Could you check a few things on this model? Use its own coordinates, in mm. Face numbers are marked on the shaded views. A direction names the side the tool comes from. Give positions to 0.01 mm unless a question says otherwise; leave off trailing zeros. Write each loop counter-clockwise with the first axis right and the second up, starting at its lowest first coordinate (ties: lowest second). Pieces come first, ordered by that corner, then holes. Notation, with made-up numbers: M 21,32 L 43,32 A20 cw 43,48 Z; hole C 40.5,22 d2. An arc over 180 degrees is marked long. Answer as a JSON object with one key per item and string values. Group by question number.
Autodesk Inventor part; units mm, degrees
ref_plane "YZ Plane" through (0, 0, 0) normal (1, 0, 0) x (0, 1, 0)
ref_plane "XZ Plane" through (0, 0, 0) normal (0, 1, 0) x (-1, 0, 0)
ref_plane "XY Plane" through (0, 0, 0) normal (0, 0, 1) x (1, 0, 0)
sketch "Skizze1" plane through (0, 0, 0) normal (0, 0, 1) x (1, 0, 0)
  line L0 (-14, 0) -> (14, 0)
  line L1 (0, -14) -> (0, 14)
  circle A0 centre (0, 0) radius 7.5
  circle A1 centre (0, 0) radius 10
  dimension "d0" = 15
  dimension "d1" = 20
extrude "Extrusion1" add sketch "Skizze1" along normal mid plane 5 contours A0 L1 A1 L0 | L0 A1 L1 A0 | A0 L0 A1 L1 | L1 A1 L0 A0
sketch "Skizze2" plane through (0, 0, 0) normal (0, 0, 1) x (1, 0, 0)
  circle A0 centre (0, 0) radius 7.5
  circle A1 centre (0, 0) radius 10
  circle A2 centre (0, 0) radius 7.5
  circle A3 centre (0, 0) radius 10
  line L0 (-14, 0) -> (14, 0)
  line L1 (0, -14) -> (0, 14)
  circle A4 centre (0, 0) radius 8.5
  dimension "d4" = 17
extrude "Extrusion2" cut sketch "Skizze2" along normal mid plane 1.5 contours A4 L1 A1 L0 | L0 A1 L1 A4 | A4 L0 A1 L1 | L1 A1 L0 A4
chamfer "Fase1" distance 1.5 angle 45 2 edges at (-10, 0, 0.75) (-10, 0, -0.75)
chamfer "Fase2" distance 0.2 angle 45 1 edges at (-7.5, 0, 2.5)
chamfer "Fase3" distance 0.2 angle 45 1 edges at (-7.5, 0, -2.5)
properties part number "Seilrolle" material "ABS-Kunststoff"
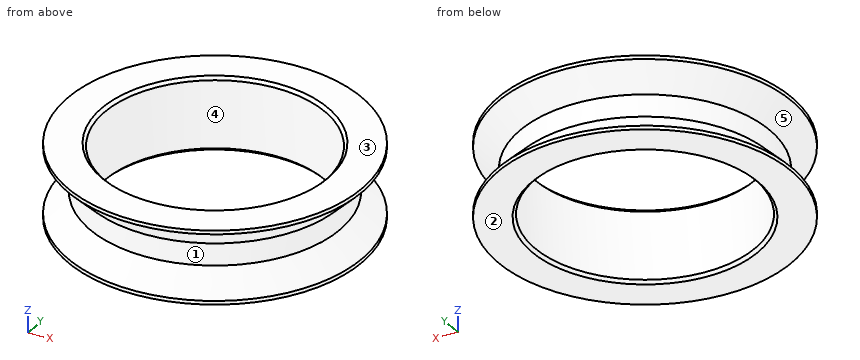
1) We'd pull the mould along Y, two halves only. Please class the marked faces 3, 4 and 5: released by +Y, released by -Y, zero draft, split by the parting line, or undercut.
2) If we section it at C-C, the plane z = -1.45: List the corners of the cut face in (x, y) for me.
3) Please list where these lines run through material, in increasing order: line 1 along X through (y, z) = (0, 0.2); line 2 along X through (y, z) = (0, -0.9). Write a range as from..to.
4) For the marked faces 1 and 2, which set-ups out of +Z, -Z, +X, -X, +Y, -Y let a thin tool reach every point of the face, with its end or its side?
5) I'm going to push a flat-ended pin straight in: pin 1 (1.5 mm diameter, centred on y = 6.5, z = 0, fed in from -X). Where does the tip first touch, or does it pass through?
Taken from the geometry:
{
 "1": {"face 3": "zero draft", "face 4": "undercut", "face 5": "split by the parting line"},
 "2": {"outline": "C 0,0 d18.4; hole C 0,0 d15"},
 "3": {"line 1": "-8.5..-7.5, 7.5..8.5", "line 2": "-8.65..-7.5, 7.5..8.65"},
 "4": {"face 1": "none", "face 2": "-Z, +X, -X, +Y, -Y"},
 "5": {"pin 1": "x = -6.26"}
}
